Part model, mm, in its own coordinate system. A direction names the side the tool comes from. Round coordinates to 2 decimals unless told otherwise and drop trailing zeros. Write each loop counter-clockwise with the first axis right and the second up, starting at its lowest first coordinate (ties: lowest second). Pieces come first, ordered by that corner, then holes. Notation, with made-up numbers: M 2.5,-36.75 L 40.5,-36.75 A13 ccw 40.5,-15.75 Z; hole C -23.5,-39 d11. An arc over 180 degrees is marked long. Use a Markdown table: item, result. Add a question column.
1) Wall check: probe 1 along X at (y, z) = (-0.75, 40.5); probe 2 along Y at (x, z) = (-26, 36.5); probe 3 along X at (y, z) = (9.5, 32). Give the ranges that are in metal, low to high.
2) Slice it at D-D on x = 42.5. Write the cut outline in (y, z), plus the area to 3 significant figures.
3) Slice it at B-B on x = 11. Write the cut outline in (y, z).
4) Which spindle directions (+Z, -Z, +X, -X, +Y, -Y) get a long thin tool onto all of the face, cutting with end or side? Do faces 5 (the face through (31.281, 8, 36)), 6 (the face through (-13.173, 13, 36)), 7 (the face through (9, 13, 29.415)). Say none if no direction does.
5) Two-plate mould, pull along Y, no slides. Class faces 1 (the face through (8, 0, 36)), 2 (the face through (29, 6, 29.326)), 3 (the face through (26.848, 5, 36)), 4 (the face through (9, 11, 36)): released by +Y, released by -Y, zero draft, split by the parting line, or undercut.
6) Slice it at C-C on z = 39.5. Write the cut outline in (x, y), plus the area to 3 significant figures.
7) Slice it at A-A on y = 6.75. Write the cut outline in (x, z), plus the area to 3 significant figures.
8) Drop flat-ended pins along their axis: P1, Ø1.1, axis at y = 0.5, z = 62, coming from the +X side; P2, Ø0.8, axis at y = 0.5, z = 62, coming from the -X side; P3, Ø8, axis at y = 6, z = 25.5, coming from the +X side. Give the stop position or say it passes through.
```python
from build123d import *

# Parameters (mm, degrees)
BOSS_EXTRUDE1_DEPTH = 1
SKETCH3_W           = 4.432871168
SKETCH3_H           = 12.941954118
BOSS_EXTRUDE4_DEPTH = 10
SKETCH4_W           = 44.453613632
SKETCH4_H           = 12.853731213
BOSS_EXTRUDE6_DEPTH = 5
CUT_EXTRUDE1_DEPTH  = 5
FILLET3_R           = 1
FILLET4_R           = 1
SKETCH7_W           = 10.96861972
SKETCH7_H           = 3.370404632
BOSS_EXTRUDE7_DEPTH = 1
SKETCH9_W           = 10.967095029
SKETCH9_H           = 3.370404632
BOSS_EXTRUDE8_DEPTH = 1


with BuildPart() as part:
    # Sketch1 → Boss-Extrude1 (new body)
    with BuildSketch(Plane(origin=(0, 0, 0), x_dir=(1, 0, 0), z_dir=(0, 1, 0))):
        with BuildLine():
            Line((76.59869755, -62.780974611), (76.937608383, -8.810873689))
            Line((76.937608383, -8.810873689), (-58.911197585, -8.810873689))
            Line((-58.911197585, -8.810873689), (-58.350110804, -62.789203863))
            ThreePointArc((-58.350110804, -62.789203863), (-57.757063466, -64.189959956), (-56.350218844, -64.768415651))
            Line((-56.350218844, -64.768415651), (74.598736982, -64.768415651))
            ThreePointArc((74.598736982, -64.768415651), (76.008503289, -64.187062528), (76.59869755, -62.780974611))
        make_face()
    extrude(amount=BOSS_EXTRUDE1_DEPTH)

    # Sketch3 → Boss-Extrude4 (add)
    with BuildSketch(Plane(origin=(0, 1, 0), x_dir=(1, 0, 0), z_dir=(0, 1, 0))):
        Polygon((-13.121429489, -42.356471833), (-8.688593239, -42.338876898), (-8.739962395, -29.397024728), (-13.172798644, -29.414619663), align=None)
        with Locations((29.064379404, -35.797373817)):
            Rectangle(SKETCH3_W, SKETCH3_H)
    extrude(amount=BOSS_EXTRUDE4_DEPTH)

    # Sketch4 → Boss-Extrude6 (add)
    with BuildSketch(Plane(origin=(0, 11, 0), x_dir=(1, 0, 0), z_dir=(0, 1, 0))):
        with Locations((9.054008172, -35.841485269)):
            Rectangle(SKETCH4_W, SKETCH4_H)
    extrude(amount=BOSS_EXTRUDE6_DEPTH)

    # Sketch5 → Cut-Extrude1 (cut)
    with BuildSketch(Plane(origin=(0, 1, 0), x_dir=(1, 0, 0), z_dir=(0, 1, 0))):
        with BuildLine():
            Line((-50.865239297, -59.658136879), (-50.865239297, -64.768415651))
            Line((-50.865239297, -64.768415651), (-46.865239297, -64.768415651))
            Line((-46.865239297, -64.768415651), (-46.865239297, -59.658136879))
            ThreePointArc((-46.865239297, -59.658136879), (-48.865239297, -57.658136879), (-50.865239297, -59.658136879))
        make_face()
        with BuildLine():
            Line((-6.748499038, -59.890356529), (-6.748499038, -64.768415651))
            Line((-6.748499038, -64.768415651), (-2.748499038, -64.768415651))
            Line((-2.748499038, -64.768415651), (-2.748499038, -59.890356529))
            ThreePointArc((-2.748499038, -59.890356529), (-4.748499038, -57.890356529), (-6.748499038, -59.890356529))
        make_face()
        with BuildLine():
            Line((65.024259069, -60.427024757), (65.024259069, -64.768415651))
            Line((65.024259069, -64.768415651), (69.024259069, -64.768415651))
            Line((69.024259069, -64.768415651), (69.024259069, -60.427024757))
            ThreePointArc((69.024259069, -60.427024757), (67.024259069, -58.427024757), (65.024259069, -60.427024757))
        make_face()
    extrude(amount=-CUT_EXTRUDE1_DEPTH, mode=Mode.SUBTRACT)

    # Fillet3
    fillet3_edges = [part.edges().sort_by_distance(p)[0] for p in [
        (9.054008172, 16, 29.414619663),
        (9.054008172, 16, 42.268350876),
    ]]
    fillet(fillet3_edges, radius=FILLET3_R)

    # Fillet4
    fillet4_edges = [part.edges().sort_by_distance(p)[0] for p in [
        (9.079535323, 11, 42.268350876),
        (9.054025631, 11, 29.414619663),
    ]]
    fillet(fillet4_edges, radius=FILLET4_R)

    # Sketch7 → Boss-Extrude7 (add)
    with BuildSketch(Plane(origin=(-58.996409176, 0, 0.613248042), x_dir=(0.010394105727731903, 0, 0.9999459798239707), z_dir=(-0.9999459798239707, 0, 0.010394105727731903))):
        with Locations((35.300658133, -0.685202316)):
            Rectangle(SKETCH7_W, SKETCH7_H)
    extrude(amount=BOSS_EXTRUDE7_DEPTH)

    # Sketch9 → Boss-Extrude8 (add)
    with BuildSketch(Plane(origin=(76.989901201, 0, 0.483466051), x_dir=(0.0062794796676542385, 0, -0.9999802838731889), z_dir=(0.9999802838731889, 0, 0.0062794796676542385))):
        with Locations((-36.296126915, -0.685202316)):
            Rectangle(SKETCH9_W, SKETCH9_H)
    extrude(amount=BOSS_EXTRUDE8_DEPTH)


solid = part.part
```
Entries:
| question | item | result |
|---|---|---|
| 1 | probe 1 | x = -59.58 to -58.58, 76.74 to 77.74 |
| 1 | probe 2 | y = 0 to 1 |
| 1 | probe 3 | x = -13.16 to -8.73, 26.85 to 31.28 |
| 2 | outline | M 0,8.81 L 1,8.81 L 1,64.77 L 0,64.77 Z |
| 2 | area | 56.0 mm^2 |
| 3 | outline | M 0,8.81 L 1,8.81 L 1,64.77 L 0,64.77 Z; M 11,30.41 A1 ccw 12,29.41 L 15,29.41 A1 ccw 16,30.41 L 16,41.27 A1 ccw 15,42.27 L 12,42.27 A1 ccw 11,41.27 Z |
| 4 | face 5 | +Z, -Z, +X, +Y |
| 4 | face 6 | +Z, -Z, -X, +Y |
| 4 | face 7 | -Z, +X, -X, +Y |
| 5 | face 1 | released by -Y |
| 5 | face 2 | zero draft |
| 5 | face 3 | undercut |
| 5 | face 4 | undercut |
| 6 | outline | M -59.59,-2.37 L -58.59,-2.37 L -58.59,0 L 76.74,0 L 76.74,-2.37 L 77.74,-2.37 L 77.74,1 L 31.28,1 L 31.28,16 L -13.17,16 L -13.17,11 L -13.13,11 L -13.13,1 L -59.59,1 Z; hole M -8.7,1 L 26.85,1 L 26.85,11 L -8.7,11 Z |
| 6 | area | 453 mm^2 |
| 7 | outline | M -13.17,29.41 L -8.74,29.4 L -8.69,42.34 L -13.12,42.36 Z; M 26.85,29.33 L 31.28,29.33 L 31.28,42.27 L 26.85,42.27 Z |
| 7 | area | 115 mm^2 |
| 8 | P1 | stops at x = 76.61 |
| 8 | P2 | stops at x = -58.36 |
| 8 | P3 | stops at x = 31.28 |
